For this review, take the finished solid that the model builds, in its own axes (mm). A direction names the side the tool comes from. Round coordinates to 2 decimals unless told otherwise and drop trailing zeros. Write each loop counter-clockwise with the first axis right and the second up, starting at its lowest first coordinate (ties: lowest second). Pieces come first, ordered by that corner, then holes. Notation, with made-up numbers: (80, 66) -> (111, 66) arc R31 cw to (111, 101) -> close; hole circle Ø11 at (-27, -9). An arc over 180 degrees is marked (long way). Answer in a Markdown table with one row per item. Add a question column.
```python
from build123d import *

# Parameters (mm, degrees)
SKETCH060_W  = 4.4
SKETCH060_H  = 4.4
PAD060_DEPTH = 0.5
SKETCH061_R  = 9.95
PAD061_DEPTH = 1.75
SKETCH059_W  = 5
SKETCH059_H  = 5
PAD059_DEPTH = 5


with BuildPart() as body059:
    # Sketch060 → Pad060 (new body)
    with BuildSketch(Plane.XZ):
        with Locations((2.2, -2.2)):
            Rectangle(SKETCH060_W, SKETCH060_H)
    extrude(amount=PAD060_DEPTH)


with BuildPart() as body059_1:
    # Body059 placement: moved
    add(body059.part.moved(Location((-2.2, 0, 2.2))))


with BuildPart() as body060:
    # Sketch061 → Pad061 (new body)
    with BuildSketch(Plane.XZ):
        Circle(SKETCH061_R)
    extrude(amount=PAD061_DEPTH)


with BuildPart() as body060_1:
    # Body060 placement: moved
    add(body060.part.moved(Location((0, -0.5, 0))))


with BuildPart() as body058:
    # Sketch059 → Pad059 (new body)
    with BuildSketch(Plane.XZ):
        with Locations((2.5, -2.5)):
            Rectangle(SKETCH059_W, SKETCH059_H)
    extrude(amount=PAD059_DEPTH)


with BuildPart() as body058_1:
    # Body058 placement: moved
    add(body058.part.moved(Location((-2, 0, 2))))


with BuildPart() as ledsimple:
    # Sphere → Sphere (revolve)
    with BuildSketch(Plane.XZ):
        with BuildLine():
            ThreePointArc((0, -1.6), (1.6, 0), (0, 1.6))
            Line((0, 1.6), (0, -1.6))
        make_face()
    revolve(axis=Axis((0, 0, 0), (0, 0, 1)))

    # Cut063: cut Body058
    add(body058_1.part, mode=Mode.SUBTRACT)

    # Fusion004: union Body059, Body060
    add(body059_1.part)
    add(body060_1.part)


with BuildPart() as ledsimple_1:
    # Fusion004 placement: moved
    add(ledsimple.part.moved(Location((0, 17, 0))))


solid = ledsimple_1.part
```
1. We need section B-B (x = 0). Write out the cut boundary in (y, z), plus the area to 3 significant figures.
2. We need section D-D (x = -8). Write out the cut boundary in (y, z).
3. We need section C-C (y = 15.35). Write out the cut boundary in (x, z), plus the area to 3 significant figures.
4. For L1, parallel to Y at x = 0, z = 8.75; L2, parallel to Y at x = 0.5, z = -2; L3, parallel to X at y = 16.55, z = -1, list the stretches that pass through material, from the lowest coordinate up. Write a range as [from, to].
5. Tool access review of faces 1 (the flat face through (0, 14.75, 0)), 2 (the flat face through (0.95, 17, 1.5)): name each direction out of +Z, -Z, +X, -X, +Y, -Y from which nothing blocks a thin tool from reaching the whole face with its end or side.
6. Clearance check with flat-ended pins moving along their axes: pin 1 Ø5 at (x, z) = (-7, 3.5) entering from +Y; pin 2 Ø1 at (y, z) = (15, 7.5) entering from +X; pin 3 Ø2 at (y, z) = (16, -4) entering from +X. State where each tip first meets the part, or that it passes through.
7. We need section A-A (z = 0). Write out the cut boundary in (x, y), plus the area to 3 significant figures.
Response:
| question | item | result |
|---|---|---|
| 1 | outline | (14.75, -9.95) -> (16.5, -9.95) -> (16.5, -2.2) -> (17, -2.2) -> (17, -1.6) arc R1.6 ccw to (17, 1.6) -> (17, 2.2) -> (16.5, 2.2) -> (16.5, 9.95) -> (14.75, 9.95) -> close |
| 1 | area | 41.0 mm2 |
| 2 | outline | (14.75, -5.92) -> (16.5, -5.92) -> (16.5, 5.92) -> (14.75, 5.92) -> close |
| 3 | outline | circle Ø19.9 at (0, 0) |
| 3 | area | 311 mm2 |
| 4 | L1 | [14.75, 16.5] |
| 4 | L2 | [14.75, 17] |
| 4 | L3 | [-2.2, 2.2] |
| 5 | face 1 | +Z, -Z, +X, -X, -Y |
| 5 | face 2 | +Y |
| 6 | pin 1 | y = 16.5 |
| 6 | pin 2 | x = 7.07 |
| 6 | pin 3 | x = 9.49 |
| 7 | outline | (-9.95, 14.75) -> (9.95, 14.75) -> (9.95, 16.5) -> (2.2, 16.5) -> (2.2, 17) -> (1.6, 17) arc R1.6 ccw to (-1.6, 17) -> (-2.2, 17) -> (-2.2, 16.5) -> (-9.95, 16.5) -> close |
| 7 | area | 41.0 mm2 |
